Can you work these out from the model? Positions are in its coordinate system, mm. A direction names the side the tool comes from. Round coordinates to 2 decimals unless told otherwise and drop trailing zeros. Loops run counter-clockwise (first coordinate to the right, second up) from the corner with the lowest first, then second, coordinate; pieces in that order, holes last.
from build123d import *

# Parameters (mm, degrees)
F4_DEPTH = 1.04


with BuildPart() as f2:
    # F1 (on Right) → F2 (revolve)
    with BuildSketch(Plane.YZ):
        with BuildLine():
            Line((-8, 0), (1.65, 0))
            Line((1.65, 0), (1.65, 2.3698039027))
            ThreePointArc((1.65, 2.3698039027), (1.1501225483, 2.7247192175), (0.55, 2.85))
            Line((0.55, 2.85), (0, 2.85))
            Line((0, 2.85), (0, 1.5))
            Line((0, 1.5), (-8, 1.5))
            Line((-8, 1.5), (-8, 0))
        make_face()
    revolve(axis=Axis((0, -3.175, 0), (0, 1, 0)))

    # F3 (on face) → F4 (cut)
    with BuildSketch(Plane(origin=(0, 1.65, 0), x_dir=(-1, 0, 0), z_dir=(0, 1, 0))):
        Polygon((-1, 0.5773502692), (-1, -0.5773502692), (0, -1.1547005384), (1, -0.5773502692), (1, 0.5773502692), (0, 1.1547005384), align=None)
    extrude(amount=-F4_DEPTH, mode=Mode.SUBTRACT)


solid = f2.part
(1) Will these pins go through, and if not, where does the flat tip stop? P1, Ø3, axis at y = -1, z = -1.5, coming from the -X side; P2, Ø3, axis at y = -5.5, z = 1.5, coming from the -X side; P3, Ø2, axis at x = 0.5, z = -0.5, coming from the +Y side; P4, Ø2, axis at y = -2, z = -1.5, coming from the -X side.
Worked answers:
P1: stops at x = -2.82
P2: stops at x = -1.5
P3: stops at y = 1.65
P4: stops at x = -1.41
(2) If we section it at A-A, the plane y = -6.25: List the corners of the cut face in (x, z) for me, then the cut area to 3 significant figures.
Worked answers:
outline: circle Ø3 at (0, 0)
area: 7.07 mm2
(3) If we mould it in two halves opening along Z, with no side actions, what happens to faces 4 (the cylindrical face through (-1.734, 0.271, -2.262)), 5 (the flat face through (0, -8, 0)), 6 (the flat face through (0, 0.61, 0))? For each: released by +Z, released by -Z, zero draft, split by the parting line, or undercut.
Worked answers:
face 4: split by the parting line
face 5: zero draft
face 6: undercut
(4) For faces 1 (the flat face through (1, 1.65, -1)), 2 (the cylindrical face through (0.07, -4.06, -1.5)), 3 (the flat face through (0.49, 1.14, 0.87)), which set-ups out of +Z, -Z, +X, -X, +Y, -Y let a thin tool reach every point of the face, with its end or its side?
Worked answers:
face 1: +Z, -Z, +X, -X, +Y
face 2: -Y
face 3: +Y
(5) If I drill on line 1 (Y direction, x = -2.25, z = 0.3); line 2 (Z direction, x = -0.1, y = -7.5), over which ranges is the centre line in solid material (lowest first)?
Worked answers:
line 1: y = 0 to 1.65
line 2: z = -1.5 to 1.5
